```python
from build123d import *

# Parameters (mm, degrees)
F0_W     = 3.175
F0_H     = 6.35
F0_H_2   = 146.05
F1_DEPTH = 101.6
F2_W     = 10.795
F2_H     = 63.5
F3_DEPTH = 3.175


with BuildPart() as f1:
    # F0 (on Top) → F1 (new body)
    with BuildSketch(Plane.XY):
        Polygon((-76.2, 76.2), (-76.2, 73.025), (-73.025, 73.025), (73.025, 73.025), (76.2, 73.025), (76.2, 76.2), align=None)
        Polygon((73.025, -31.75), (73.025, -73.025), (76.2, -73.025), (76.2, -41.275), (76.2, -38.1), (76.2, -31.75), align=None)
        with Locations((82.2325, 34.925)):
            Rectangle(F0_W, F0_H)
        Polygon((-73.025, -73.025), (-76.2, -73.025), (-76.2, -76.2), (76.2, -76.2), (76.2, -73.025), (73.025, -73.025), align=None)
        Polygon((76.2, -38.1), (76.2, -41.275), (83.82, -41.275), (83.82, -38.1), (80.645, -38.1), align=None)
        with Locations((82.2325, -34.925)):
            Rectangle(F0_W, F0_H)
        Polygon((76.2, 73.025), (73.025, 73.025), (73.025, 31.75), (76.2, 31.75), (76.2, 38.1), (76.2, 41.275), align=None)
        Polygon((83.82, 41.275), (76.2, 41.275), (76.2, 38.1), (80.645, 38.1), (83.82, 38.1), align=None)
        with Locations((-74.6125, 0)):
            Rectangle(F0_W, F0_H_2)
    extrude(amount=F1_DEPTH)

    # F2 (on Top) → F3 (join)
    with BuildSketch(Plane.XY):
        Polygon((73.025, 31.75), (73.025, 73.025), (-73.025, 73.025), (-73.025, -73.025), (73.025, -73.025), (73.025, -31.75), align=None)
        with Locations((78.4225, 0)):
            Rectangle(F2_W, F2_H)
    extrude(amount=F3_DEPTH)


solid = f1.part
```
Check sheet for the modelled part. Datum: model origin and axes. Units: mm. A direction names the side the tool comes from. Round coordinates to 2 decimals unless told otherwise and drop trailing zeros. Loops run counter-clockwise (first coordinate to the right, second up) from the corner with the lowest first, then second, coordinate; pieces in that order, holes last. Notation, with made-up numbers: (20.25, -35) - (65.25, -35) arc R18 cw to (65.25, -9) - close; hole circle Ø1 at (13.5, 6). An arc over 180 degrees is marked (long way). Answer as a JSON object with one key per item and string values. Group by question number.
Q1. Scan lines: line 1 along X through (y, z) = (36, 70) (3 decimals); line 2 along X through (y, z) = (-65.5, 60) (3 decimals). Record each from-to range of solid material in increasing order. Write a range as [from, to].
Q2. Set-up check for faces 1 (the face through (76.2, 58, 50)), 2 (the face through (76.2, -35, 50)), 3 (the face through (-8, 74, 101.6)), 4 (the face through (3, 1, 0)), 5 (the face through (-1, 73.025, 52)): record each of +Z, -Z, +X, -X, +Y, -Y from which the full face is reachable in a straight line by a thin tool's end or side.
Q3. Mould release check, pull along X, two halves, no side actions. Record for faces 6 (the face through (1, 76.2, 50)), 7 (the face through (73.025, -52, 52)), 8 (the face through (-76.2, 1, 50)): released by +X, released by -X, zero draft, split by the parting line, or undercut.
Q4. Gauge pin test, flat ends, axial feed: P1, Ø1.6, axis at x = 79.5, z = 1, coming from the -Y side (3 decimals); P2, Ø2.5, axis at x = 81.5, z = 74, coming from the +Y side (3 decimals); P3, Ø5, axis at x = -10, y = 28.5, coming from the +Z side (3 decimals). Record the tip position at first contact, or that the pin passes through.
Q5. Sectioned sample at D-D, the plane y = 12. Enter the section's corners in (x, z) (3 decimals), plus the area to 3 significant figures.
Q6. Sectioned sample at A-A, the plane z = 17. Enter the section's corners in (x, y) (3 decimals), plus the area to 3 significant figures.
Q7. Sectioned sample at B-B, the plane y = 57. Enter the section's corners in (x, z) (3 decimals), plus the area to 3 significant figures.
Solution:
{
 "1": {"line 1": "x = [-76.2, -73.025], [73.025, 76.2], [80.645, 83.82]", "line 2": "x = [-76.2, -73.025], [73.025, 76.2]"},
 "2": {"face 1": "+Z, -Z, +X, +Y", "face 2": "+Z, -Z", "face 3": "+Z, +X, -X, +Y, -Y", "face 4": "-Z, +X, -X, +Y, -Y", "face 5": "+Z"},
 "3": {"face 6": "zero draft", "face 7": "undercut", "face 8": "released by -X"},
 "4": {"P1": "stops at y = -41.275", "P2": "stops at y = 41.275", "P3": "stops at z = 3.175"},
 "5": {"outline": "(-76.2, 0) - (83.82, 0) - (83.82, 3.175) - (-73.025, 3.175) - (-73.025, 101.6) - (-76.2, 101.6) - close", "area": "821 mm²"},
 "6": {"outline": "(-76.2, -76.2) - (76.2, -76.2) - (76.2, -41.275) - (83.82, -41.275) - (83.82, -31.75) - (80.645, -31.75) - (80.645, -38.1) - (76.2, -38.1) - (76.2, -31.75) - (73.025, -31.75) - (73.025, -73.025) - (-73.025, -73.025) - (-73.025, 73.025) - (73.025, 73.025) - (73.025, 31.75) - (76.2, 31.75) - (76.2, 38.1) - (80.645, 38.1) - (80.645, 31.75) - (83.82, 31.75) - (83.82, 41.275) - (76.2, 41.275) - (76.2, 76.2) - (-76.2, 76.2) - close", "area": "1,780 mm²"},
 "7": {"outline": "(-76.2, 0) - (76.2, 0) - (76.2, 101.6) - (73.025, 101.6) - (73.025, 3.175) - (-73.025, 3.175) - (-73.025, 101.6) - (-76.2, 101.6) - close", "area": "1,110 mm²"}
}
